Autodesk Inventor part; units mm, degrees
ref_plane "YZ Plane" through (0, 0, 0) normal (1, 0, 0) x (0, 1, 0)
ref_plane "XZ Plane" through (0, 0, 0) normal (0, 1, 0) x (-1, 0, 0)
ref_plane "XY Plane" through (0, 0, 0) normal (0, 0, 1) x (1, 0, 0)
sketch "Sketch1" plane through (0, 0, 0) normal (0, 0, 1) x (1, 0, 0)
  line L0 (-16.019, 0) -> (21.981, 0)
  line L1 (-16.019, 1.5) -> (21.681, 1.5)
  line L2 (-16.019, 0) -> (-16.019, 2.85)
  line L3 (-17.669, 0) -> (-17.669, 1.425)
  line L4 (21.981, 1.2) -> (21.981, 0)
  line L5 (-16.369, 0) -> (-16.369, 2.85)
  line L6 (-16.019, 2.85) -> (-16.369, 2.85)
  arc A0 (-16.369, 2.85) -> (-17.669, 1.425) centre (-14.6489, -0.0247) ccw
  line L7 (21.681, 1.5) -> (21.981, 1.2)
  line L8 (-16.019, 0) -> (-17.669, 0)
  point P0 (0, 0)
  point P1 (21.981, 1.5)
  dimension "d0" = 38
  dimension "d1" = 1.5
  dimension "d2" = 2.85
  dimension "d3" = 1.425
  dimension "d4" = 1.65
  dimension "d5" = 2.85
  dimension "d6" = 0.35
  dimension "d7" = 3.35
  dimension "d8" = 0.3
  dimension "d9" = 45
revolve "Revolution1" add sketch "Sketch1" angle 360 about axis through (-16.019, 0, 0) along (1, 0, 0)
sketch "Sketch2" plane through (-17.669, 0, 0) normal (-1, 0, 0) x (0, 0, 1)
  line L0 (-1, 0) -> (-0.5, 0.866)
  line L1 (-0.5, 0.866) -> (0.5, 0.866)
  line L2 (0.5, 0.866) -> (1, 0)
  line L3 (1, 0) -> (0.5, -0.866)
  line L4 (0.5, -0.866) -> (-0.5, -0.866)
  line L5 (-0.5, -0.866) -> (-1, 0)
  point P0 (0, 0)
  point P1 (0, 0)
  dimension "d11" = 2
extrude "Extrusion1" cut sketch "Sketch2" against normal blind 1
thread "Thread1"
properties part number "bolt" material "Steel, Mild, Welded"
Input: part model. Units: mm. Frame: model coordinates. A direction names the side the tool comes from. Give positions to 0.01 mm unless a question says otherwise; leave off trailing zeros. Order: outer loops, then holes, each group sorted by start corner. A loop starts at its lowest first (then second) coordinate and runs counter-clockwise, first axis right, second up. Notation, with made-up numbers: M 14.25,30 L 38.25,30 A21 ccw 38.25,65 Z; hole C 42,50 d8. An arc over 180 degrees is marked long. Answer as a JSON object with one key per item and string values.
1. Reachability of faces 1 (the cylindrical face through (3.09, -1.5, 0.07)), 2 (the flat face through (21.981, 0, 0)), 3 (the flat face through (-17.18, 0.43, -0.75)) from +Z, -Z, +X, -X, +Y, -Y: full face, straight path, thin tool, end or side. Return the list, or none.
Result sheet:
{"face 1": "+X", "face 2": "+Z, -Z, +X, +Y, -Y", "face 3": "-X"}
2. Pull-direction query (Y, two-part tool) for faces 4 (the cylindrical face through (-16.196, -2.262, 1.734)), 5 (the flat face through (-17.176, -0.439, -0.746)), 6 (the flat face through (-16.669, 0, 0)), 7 (the flat face through (-16.019, 1.2, -1.2)); classes: +Y half, -Y half, draft (parallel to the pull), parting line (faces both ways), or undercut.
Result sheet:
{"face 4": "parting line", "face 5": "undercut", "face 6": "undercut", "face 7": "draft"}
3. First-contact query: P1, Ø2, axis at x = -9.5, y = 0.5, coming from the +Z side; P2, Ø1.9, axis at y = 0, z = 0.5, coming from the -X side; P3, Ø2, axis at x = 12, y = 0, coming from the -Z side; P4, Ø1.5, axis at x = 10, z = 1.5, coming from the -Y side. Flat tips, straight axial feed; report the tip coordinate or a pass-through.
Result sheet:
{"P1": "z = 1.5", "P2": "x = -17.67", "P3": "z = -1.5", "P4": "y = -1.3"}
4. Cut plane A-A, the plane x = -15. Output: boundary loops of the cut face in (y, z), and give its area (3 significant figures).
Result sheet:
{"outline": "C 0,0 d3", "area": "7.07 mm²"}
5. Ray query, line 1 (X direction, y = -0.5, z = -0.15); line 2 (Y direction, x = -15, z = -0.9); line 3 (Y direction, x = 4.5, z = 0.1). Return the intervals inside material, ascending. Write a range as [from, to].
Result sheet:
{"line 1": "[-16.67, 21.98]", "line 2": "[-1.2, 1.2]", "line 3": "[-1.5, 1.5]"}
